Can you work these out from the model? Positions are in its coordinate system, mm. A direction names the side the tool comes from. Round coordinates to 2 decimals unless told otherwise and drop trailing zeros. Write each loop counter-clockwise with the first axis right and the second up, starting at its lowest first coordinate (ties: lowest second). Pieces come first, ordered by that corner, then holes. Notation, with made-up numbers: M 36,8.25 L 51,8.25 A21 ccw 51,29.25 Z; hole C -10.5,-1.5 d7. An arc over 180 degrees is marked long. Answer in a Markdown table with one row per item. Add a question column.
(1) I'm going to push flat-ended pins straight in: pin 1 (6 mm diameter, centred on x = 0, z = 62.5, fed in from +Y); pin 2 (8 mm diameter, centred on x = -41, z = -42.5, fed in from -Y); pin 3 (3 mm diameter, centred on x = -7, y = 4, fed in from +Z); pin 4 (4 mm diameter, centred on y = 7.5, z = -31, fed in from +X). Where does each tip first touch, or does it pass through?
(2) Suppose I cut it at B-B, the plane z = 0. Write out the boundary of the cut face in (x, y).
(3) If I drill on probe 1 along Y at (x, z) = (47.5, -46); probe 2 along X at (y, z) = (6.25, 5.5); probe 3 along X at (y, z) = (3.05, -62.5), over which ranges is the centre line in solid material (lowest first)?
(4) If we mould it in two halves opening along Z, with no side actions, what happens to faces 3 (the face through (-46.245, 2.465, -60.311)), 4 (the face through (-68, 10, -3.25)), 5 (the face through (-68, 15, -8))? For each: released by +Z, released by -Z, zero draft, split by the parting line, or undercut.
(5) Suppose I cut it at A-A, the plane x = 0. Write out the boundary of the cut face in (y, z).
(6) Suppose I cut it at C-C, the plane z = -62.5. Write out the boundary of the cut face in (x, y).
(7) For faces 1 (the face through (68, 15, 8)), 2 (the face through (67, 10, 13.25)), which set-ups out of +Z, -Z, +X, -X, +Y, -Y let a thin tool reach every point of the face, with its end or its side?
(8) Suppose I cut it at D-D, the plane x = 66.5. Write out the boundary of the cut face in (y, z), then the cut area to 3 significant figures.
from build123d import *

# Parameters (mm, degrees)
SKETCH1_R           = 76
SKETCH1_W           = 100
SKETCH1_H           = 100
BOSS_EXTRUDE1_DEPTH = 5
SKETCH3_W           = 100
SKETCH3_H           = 100
BOSS_EXTRUDE2_DEPTH = 5
SKETCH3_2_W         = 100
SKETCH3_2_H         = 100
CUT_EXTRUDE1_DEPTH  = 2
SKETCH6_R           = 2.25
CUT_EXTRUDE2_DEPTH  = 10
SKETCH8_R           = 73
SKETCH8_R_2         = 70.710678119
BOSS_EXTRUDE3_DEPTH = 5
BOSS_EXTRUDE4_DEPTH = 10
BOSS_EXTRUDE5_DEPTH = 5
BOSS_EXTRUDE7_DEPTH = 10
BOSS_EXTRUDE8_DEPTH = 5
CUT_EXTRUDE3_DEPTH  = 27
CUT_EXTRUDE4_DEPTH  = 27


with BuildPart() as part:
    # Sketch1 → Boss-Extrude1 (new body)
    with BuildSketch(Plane(origin=(0, 0, 0), x_dir=(1, 0, 0), z_dir=(0, 1, 0))):
        with Locations(Location((0, 0, 0), (0, 0, 270))):
            Circle(SKETCH1_R)
        Rectangle(SKETCH1_W, SKETCH1_H, mode=Mode.SUBTRACT)
    extrude(amount=BOSS_EXTRUDE1_DEPTH)

    # Sketch3 → Boss-Extrude2 (add)
    with BuildSketch(Plane(origin=(0, 5, 0), x_dir=(1, 0, 0), z_dir=(0, 1, 0))):
        Rectangle(SKETCH3_W, SKETCH3_H)
    extrude(amount=-BOSS_EXTRUDE2_DEPTH)

    # Sketch3_2 → Cut-Extrude1 (cut)
    with BuildSketch(Plane(origin=(0, 5, 0), x_dir=(1, 0, 0), z_dir=(0, 1, 0))):
        Rectangle(SKETCH3_2_W, SKETCH3_2_H)
    extrude(amount=-CUT_EXTRUDE1_DEPTH, mode=Mode.SUBTRACT)

    # Sketch6 → Cut-Extrude2 (cut)
    with BuildSketch(Plane(origin=(0, 5, 0), x_dir=(1, 0, 0), z_dir=(0, 1, 0))):
        with Locations(Location((0, 62.5, 0), (0, 0, 270))):
            Circle(SKETCH6_R)
        with Locations(Location((62.5, 0, 0), (0, 0, 270))):
            Circle(SKETCH6_R)
        with Locations(Location((0, -62.5, 0), (0, 0, 270))):
            Circle(SKETCH6_R)
        with Locations(Location((-62.5, 0, 0), (0, 0, 270))):
            Circle(SKETCH6_R)
    extrude(amount=-CUT_EXTRUDE2_DEPTH, mode=Mode.SUBTRACT)

    # Sketch8 → Boss-Extrude3 (add)
    with BuildSketch(Plane(origin=(0, 5, 0), x_dir=(1, 0, 0), z_dir=(0, 1, 0))):
        with Locations(Location((0, 0, 0), (0, 0, 270))):
            Circle(SKETCH8_R)
        with Locations(Location((0, 0, 0), (0, 0, 135))):
            Circle(SKETCH8_R_2, mode=Mode.SUBTRACT)
    extrude(amount=BOSS_EXTRUDE3_DEPTH)

    # Sketch11 → Boss-Extrude4 (add)
    with BuildSketch(Plane(origin=(0, 5, 0), x_dir=(1, 0, 0), z_dir=(0, 1, 0))):
        with BuildLine():
            Line((70.635950478, -3.25), (62.5, -3.25))
            Line((62.5, -3.25), (62.5, -13.25))
            Line((62.5, -13.25), (69.458170866, -13.25))
            ThreePointArc((69.458170866, -13.25), (70.225285395, -8.270990945), (70.635950478, -3.25))
        make_face()
    extrude(amount=BOSS_EXTRUDE4_DEPTH)

    # Sketch12 → Boss-Extrude5 (add)
    with BuildSketch(Plane(origin=(0, 10, 0), x_dir=(1, 0, 0), z_dir=(0, 1, 0))):
        with BuildLine():
            Line((72.927618225, -3.25), (70.635950478, -3.25))
            ThreePointArc((70.635950478, -3.25), (70.225285395, -8.270990945), (69.458170866, -13.25))
            Line((69.458170866, -13.25), (71.787446674, -13.25))
            ThreePointArc((71.787446674, -13.25), (72.530079982, -8.269673379), (72.927618225, -3.25))
        make_face()
    extrude(amount=BOSS_EXTRUDE5_DEPTH)

    # Sketch13 → Boss-Extrude7 (add)
    with BuildSketch(Plane(origin=(0, 5, 0), x_dir=(1, 0, 0), z_dir=(0, 1, 0))):
        with BuildLine():
            Line((-70.635950478, 3.25), (-62.5, 3.25))
            Line((-62.5, 3.25), (-62.5, 13.25))
            Line((-62.5, 13.25), (-69.458170866, 13.25))
            ThreePointArc((-69.458170866, 13.25), (-70.225285395, 8.270990945), (-70.635950478, 3.25))
        make_face()
    extrude(amount=BOSS_EXTRUDE7_DEPTH)

    # Sketch14 → Boss-Extrude8 (add)
    with BuildSketch(Plane(origin=(0, 10, 0), x_dir=(1, 0, 0), z_dir=(0, 1, 0))):
        with BuildLine():
            Line((-69.458170866, 13.25), (-71.787446674, 13.25))
            ThreePointArc((-71.787446674, 13.25), (-72.530079982, 8.269673379), (-72.927618225, 3.25))
            Line((-72.927618225, 3.25), (-70.635950478, 3.25))
            ThreePointArc((-70.635950478, 3.25), (-70.225285395, 8.270990945), (-69.458170866, 13.25))
        make_face()
    extrude(amount=BOSS_EXTRUDE8_DEPTH)

    # Sketch17 → Cut-Extrude3 (cut)
    with BuildSketch(Plane(origin=(-62.5, 0, 0), x_dir=(0, 0, -1), z_dir=(1, 0, 0))):
        with BuildLine():
            ThreePointArc((8.25, 11.5), (6.75, 10), (8.25, 8.5))
            Line((8.25, 8.5), (8.25, 11.5))
        make_face()
        with BuildLine():
            Line((8.25, 11.5), (8.25, 8.5))
            ThreePointArc((8.25, 8.5), (9.310660172, 8.939339828), (9.75, 10))
            ThreePointArc((9.75, 10), (9.310660172, 11.060660172), (8.25, 11.5))
        make_face()
    extrude(amount=-CUT_EXTRUDE3_DEPTH, mode=Mode.SUBTRACT)

    # Sketch18 → Cut-Extrude4 (cut)
    with BuildSketch(Plane.ZY.offset(-62.5)):
        with BuildLine():
            ThreePointArc((9.75, 10), (9.310660172, 11.060660172), (8.25, 11.5))
            Line((8.25, 11.5), (8.25, 8.5))
            ThreePointArc((8.25, 8.5), (9.310660172, 8.939339828), (9.75, 10))
        make_face()
        with BuildLine():
            Line((8.25, 8.5), (8.25, 11.5))
            ThreePointArc((8.25, 11.5), (6.75, 10), (8.25, 8.5))
        make_face()
    extrude(amount=-CUT_EXTRUDE4_DEPTH, mode=Mode.SUBTRACT)


solid = part.part
Calculated:
| question | item | result |
|---|---|---|
| 1 | pin 1 | y = 5 |
| 1 | pin 2 | y = 0 |
| 1 | pin 3 | z = 75.8 |
| 1 | pin 4 | x = 66.99 |
| 2 | outline | M -76,0 L -64.75,0 L -64.75,5 L -70.71,5 L -70.71,10 L -73,10 L -73,5 L -76,5 Z; M -60.25,0 L 60.25,0 L 60.25,5 L 50,5 L 50,3 L -50,3 L -50,5 L -60.25,5 Z; M 64.75,0 L 76,0 L 76,5 L 73,5 L 73,10 L 70.71,10 L 70.71,5 L 64.75,5 Z |
| 3 | probe 1 | 0 to 3 |
| 3 | probe 2 | -72.79 to -70.5, 62.5 to 72.79 |
| 3 | probe 3 | -43.24 to -2.25, 2.25 to 43.24 |
| 4 | face 3 | split by the parting line |
| 4 | face 4 | undercut |
| 4 | face 5 | zero draft |
| 5 | outline | M 0,-76 L 5,-76 L 5,-73 L 10,-73 L 10,-70.71 L 5,-70.71 L 5,-64.75 L 0,-64.75 Z; M 0,-60.25 L 5,-60.25 L 5,-50 L 3,-50 L 3,50 L 5,50 L 5,60.25 L 0,60.25 Z; M 0,64.75 L 5,64.75 L 5,70.71 L 10,70.71 L 10,73 L 5,73 L 5,76 L 0,76 Z |
| 6 | outline | M -43.24,0 L -2.25,0 L -2.25,5 L -33.07,5 L -33.07,10 L -37.72,10 L -37.72,5 L -43.24,5 Z; M 2.25,0 L 43.24,0 L 43.24,5 L 37.72,5 L 37.72,10 L 33.07,10 L 33.07,5 L 2.25,5 Z |
| 7 | face 1 | +Z, -Z, +X, -X, +Y |
| 7 | face 2 | +Y |
| 8 | outline | M 0,-36.79 L 5,-36.79 L 5,-30.11 L 10,-30.11 L 10,-24.04 L 5,-24.04 L 5,3.25 L 15,3.25 L 15,13.25 L 5,13.25 L 5,24.04 L 10,24.04 L 10,30.11 L 5,30.11 L 5,36.79 L 0,36.79 Z; hole C 10,8.25 d3 |
| 8 | area | 522 mm² |
